from build123d import *

# Parameters (mm, degrees)
F0_W     = 60.493108
F0_H     = 50.502148
F1_DEPTH = 127.8868
F3_DEPTH = 76.2


with BuildPart() as f1:
    # F0 (on Top) → F1 (new body)
    with BuildSketch(Plane.XY):
        with Locations((30.246554, 25.251074)):
            Rectangle(F0_W, F0_H)
    extrude(amount=F1_DEPTH)

    # F2 (on face) → F3 (join)
    with BuildSketch(Plane.XZ):
        Polygon((35.168027, 80.730942), (38.657124, 82.189071), (41.766813, 84.34076), (44.361187, 87.091971), (46.326859, 90.322462), (47.57792, 93.891045), (48.059691, 97.641756), (47.751118, 101.410671), (46.665687, 105.03307), (44.850836, 108.350637), (42.385883, 111.218379), (39.378557, 113.510961), (35.960295, 115.128186), (32.28049, 115.999375), (28.499966, 116.086451), (24.783953, 115.38561), (21.294856, 113.927481), (18.185166, 111.775791), (15.590792, 109.024581), (13.62512, 105.79409), (12.37406, 102.225507), (11.892288, 98.474796), (12.200861, 94.705881), (13.286293, 91.083482), (15.101144, 87.765915), (17.566097, 84.898173), (20.573422, 82.605591), (23.991685, 80.988365), (27.67149, 80.117177), (31.452013, 80.030101), align=None)
        Polygon((35.833944, 13.889787), (41.954983, 16.244033), (47.048936, 20.374559), (50.617169, 25.877041), (52.310401, 32.212857), (51.962885, 38.761813), (49.608639, 44.882853), (45.478113, 49.976805), (39.975631, 53.545039), (33.639815, 55.238271), (27.090859, 54.890755), (20.969819, 52.536509), (15.875867, 48.405983), (12.307633, 42.903501), (10.614401, 36.567685), (10.961917, 30.018728), (13.316163, 23.897689), (17.446689, 18.803736), (22.949171, 15.235502), (29.284987, 13.542271), align=None)
    extrude(amount=F3_DEPTH)


solid = f1.part
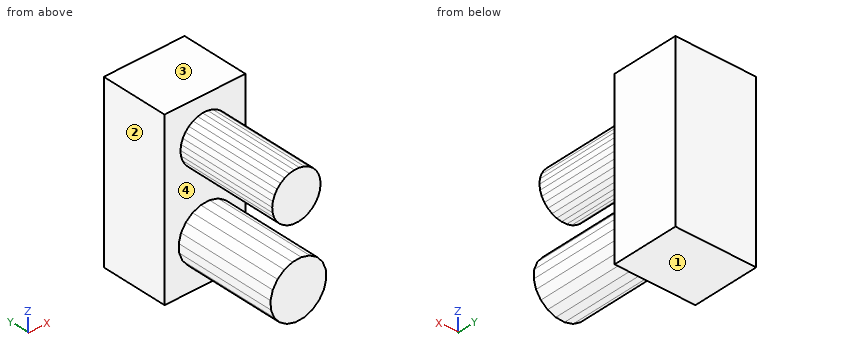
Check sheet for the modelled part. Datum: model origin and axes. Units: mm. Face numbers are marked on the shaded views. Round coordinates to 2 decimals unless told otherwise and drop trailing zeros. Loops run counter-clockwise (first coordinate to the right, second up) from the corner with the lowest first, then second, coordinate; pieces in that order, holes last.
1. Sectioned sample at A-A on x = 5. Record the boundary of the cut face in (y, z), and give its area (3 significant figures).
2. Sectioned sample at B-B on z = 118. Record the boundary of the cut face in (x, y), and give its area (3 significant figures).
3. Mould release check, pull along Z, two halves, no side actions. Record for the marked faces 1, 2, 3 and 4: released by +Z, released by -Z, zero draft, split by the parting line, or undercut.
4. Scan lines: probe 1 along Y at (x, z) = (8, 22.5); probe 2 along Z at (x, y) = (17, -5); probe 3 along Z at (x, y) = (28.5, -23). Record each from-to range of solid material in increasing order.
5. Gauge pin test, flat ends, axial feed: pin 1 Ø4 at (y, z) = (0.5, 40) entering from -X; pin 2 Ø10 at (y, z) = (-57, 78) entering from +X; pin 3 Ø3 at (x, z) = (12.5, 82.5) entering from -Y; pin 4 Ø8 at (x, y) = (35, -44) entering from +Z. Record the tip position at first contact, or that the pin passes through.
Recorded:
1. outline: (0, 0) - (50.5, 0) - (50.5, 127.89) - (0, 127.89) - close
1. area: 6,460 mm2
2. outline: (0, 0) - (60.49, 0) - (60.49, 50.5) - (0, 50.5) - close
2. area: 3,060 mm2
3. face 1: released by -Z
3. face 2: zero draft
3. face 3: released by +Z
3. face 4: undercut
4. probe 1: y = 0 to 50.5
4. probe 2: z = 19.35 to 49.32, 85.56 to 110.52
4. probe 3: z = 13.75 to 54.97, 80.1 to 116.09
5. pin 1: stops at x = 0
5. pin 2: stops at x = 39.83
5. pin 3: stops at y = 0
5. pin 4: stops at z = 116.03
